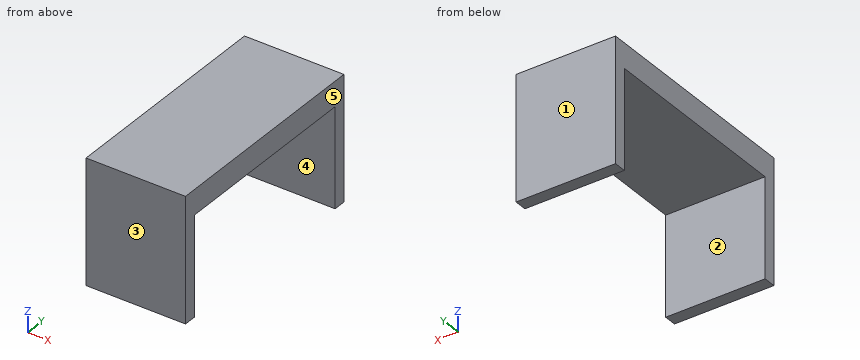
from build123d import *

# Parameters (mm, degrees)
F0_W     = 25.4
F0_H     = 3.175
F0_H_2   = 50.8
F1_DEPTH = 31.75
F2_DEPTH = 25.4


with BuildPart() as f1:
    # F0 (on Top) → F1 (new body)
    with BuildSketch(Plane.XY):
        with Locations((-16.626253, 23.70746)):
            Rectangle(F0_W, F0_H)
        with Locations((-16.626253, -3.28004)):
            Rectangle(F0_W, F0_H_2)
        with Locations((-16.626253, -30.26754)):
            Rectangle(F0_W, F0_H)
    extrude(amount=F1_DEPTH)

    # F0 (on Top) → F2 (cut)
    with BuildSketch(Plane.XY):
        with Locations((-16.626253, -3.28004)):
            Rectangle(F0_W, F0_H_2)
    extrude(amount=F2_DEPTH, mode=Mode.SUBTRACT)


solid = f1.part
Source: CAD feature listing. Evaluate the final solid. Frame: model axes, mm. Face numbers are marked on the shaded views. A direction names the side the tool comes from. Coordinates: 2 decimals unless noted, no trailing zeros. Loops run counter-clockwise (first coordinate to the right, second up) from the corner with the lowest first, then second, coordinate; pieces in that order, holes last. Notation, with made-up numbers: (74.25, 35.25) - (107.25, 35.25) arc R8 cw to (107.25, 48.25) - close; hole circle Ø8 at (-15, -17.5). An arc over 180 degrees is marked (long way). Return JSON: item names as keys, results as strings.
Q1. Mould query, pull axis Y, two halves, no side actions, for the marked faces 1, 2 and 3. Classes: released by +Y, released by -Y, zero draft, split by the parting line, or undercut.
Results:
{"face 1": "released by +Y", "face 2": "undercut", "face 3": "released by -Y"}
Q2. Section B-B, the plane x = -24.25. Return loops of the section in (y, z), plus the area to 3 significant figures.
Results:
{"outline": "(-31.86, 0) - (-28.68, 0) - (-28.68, 25.4) - (22.12, 25.4) - (22.12, 0) - (25.29, 0) - (25.29, 31.75) - (-31.86, 31.75) - close", "area": "524 mm2"}
Q3. Section C-C, the plane y = -21. Return loops of the section in (x, z).
Results:
{"outline": "(-29.33, 25.4) - (-3.93, 25.4) - (-3.93, 31.75) - (-29.33, 31.75) - close"}
Q4. Section A-A, the plane z = 2. Return loops of the section in (x, y), plus the area to 3 significant figures.
Results:
{"outline": "(-29.33, -31.86) - (-3.93, -31.86) - (-3.93, -28.68) - (-29.33, -28.68) - close; (-29.33, 22.12) - (-3.93, 22.12) - (-3.93, 25.29) - (-29.33, 25.29) - close", "area": "161 mm2"}
Q5. Access query for the marked faces 4 and 5. Directions: +Z, -Z, +X, -X, +Y, -Y. A direction counts if a zero-diameter tool reaches every point of the face in a straight line with its end or side. Return the directions, or none.
Results:
{"face 4": "-Z, +X, -X", "face 5": "+Z, -Z, +X, +Y, -Y"}
Q6. Contact query for flat-ended pins moving along their axis: P1, Ø4, axis at y = -25, z = 7, coming from the +X side; P2, Ø2, axis at x = -26, y = -22.5, coming from the -Z side. Output: stop coordinate, or through.
Results:
{"P1": "through", "P2": "z = 25.4"}
Q7. Material intervals for line 1 along Y through (x, z) = (-11.75, 21); line 2 along Z through (x, y) = (-16.5, 14.5), sorted ascending.
Results:
{"line 1": "-31.86 to -28.68, 22.12 to 25.29", "line 2": "25.4 to 31.75"}
